Source: three-view drawing plus pictorial views. Frame: mm from the lowest corner of the part. A direction names the side the tool comes from. Give positions to 0.01 mm unless a question says otherwise; leave off trailing zeros. Loops run counter-clockwise (first coordinate to the right, second up) from the corner with the lowest first, then second, coordinate; pieces in that order, holes last.
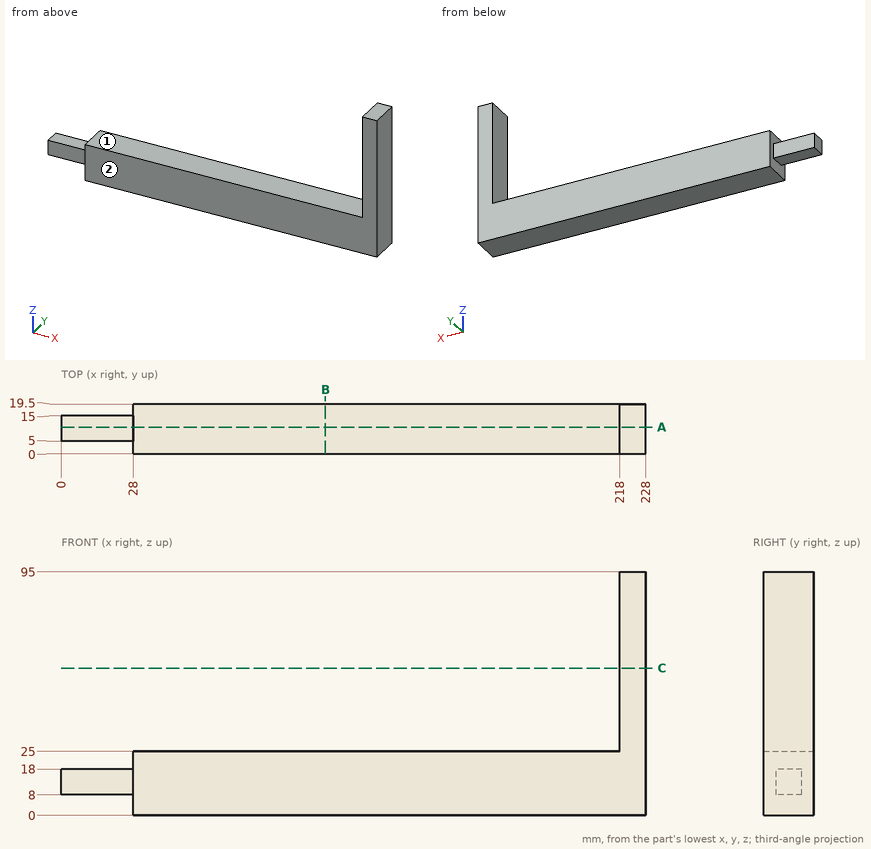
1) Cut plane A-A (y = 10.5). Return loops of the section in (x, z), and give its area (3 significant figures).
Checks:
outline: (0, 8) - (28, 8) - (28, 0) - (228, 0) - (228, 95) - (218, 95) - (218, 25) - (28, 25) - (28, 18) - (0, 18) - close
area: 5,980 mm2
2) Reachability of the marked faces 1 and 2 from +Z, -Z, +X, -X, +Y, -Y: full face, straight path, thin tool, end or side. Return the list, or none.
Checks:
face 1: +Z, -X, +Y, -Y
face 2: +Z, -Z, +X, -X, -Y
3) Ray query, probe 1 along X at (y, z) = (15.75, 78.5); probe 2 along Z at (x, y) = (35, 12.5); probe 3 along X at (y, z) = (7.75, 6). Return the intervals inside material, ascending.
Checks:
probe 1: x = 218 to 228
probe 2: z = 0 to 25
probe 3: x = 28 to 228
4) Cut plane B-B (x = 103). Return loops of the section in (y, z).
Checks:
outline: (0, 0) - (19.5, 0) - (19.5, 25) - (0, 25) - close
5) Cut plane C-C (z = 57.5). Return loops of the section in (x, y).
Checks:
outline: (218, 0) - (228, 0) - (228, 19.5) - (218, 19.5) - close
6) Contact query for flat-ended pins moving along their axis: P1, Ø5, axis at x = 15.5, y = 9.5, coming from the +Z side; P2, Ø3, axis at x = 10.5, z = 15, coming from the +Y side; P3, Ø3, axis at x = 20, z = 12, coming from the -Y side. Output: stop coordinate, or through.
Checks:
P1: stops at z = 18
P2: stops at y = 15
P3: stops at y = 5
